Source: CAD feature listing. Evaluate the final solid. Frame: model axes, mm. Face numbers are marked on the shaded views. Give positions to 0.01 mm unless a question says otherwise; leave off trailing zeros. Order: outer loops, then holes, each group sorted by start corner. A loop starts at its lowest first (then second) coordinate and runs counter-clockwise, first axis right, second up. Notation, with made-up numbers: M 9.25,4.25 L 35.25,4.25 A23 ccw 35.25,23.25 Z; hole C -31.5,-14.75 d8. An arc over 180 degrees is marked long. Use CSV: the item, a comma, the result in double quotes. Start each with the question number.
1. Mould query, pull axis X, two halves, no side actions, for the marked faces 1, 2, 3 and 4. Classes: released by +X, released by -X, zero draft, split by the parting line, or undercut.
2. Section query A-A, the plane x = 0. Return the cut outline in (y, z), plus the area to 3 significant figures.
3. Section query C-C, the plane z = -9. Return the cut outline in (x, y).
4. Line query: line 1 along Y through (x, z) = (0, -2); line 2 along Y through (x, z) = (12, -6); line 3 along X through (y, z) = (17, 18.5). Output: solid intervals per line, ascending. Write a range as [from, to].
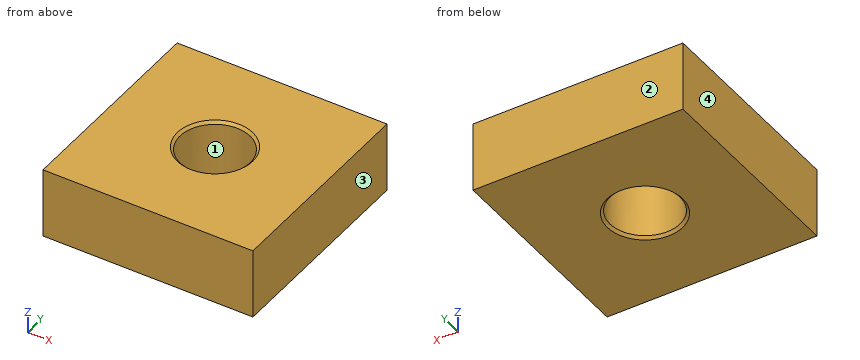
from build123d import *

# Parameters (mm, degrees)
SKETCH1_W          = 120
SKETCH1_H          = 120
SKETCH1_R          = 20
EXTRUDE1_DEPTH     = 20
FRAME_CHAMFER_SIZE = 1.5


with BuildPart() as part:
    # Sketch1 → Extrude1 (new body, symmetric)
    with BuildSketch(Plane.XY):
        Rectangle(SKETCH1_W, SKETCH1_H)
        Circle(SKETCH1_R, mode=Mode.SUBTRACT)
    extrude(amount=EXTRUDE1_DEPTH, both=True)

    # Frame Chamfer
    frame_chamfer_edges = [part.edges().sort_by_distance(p)[0] for p in [
        (-20, 0, -20),
        (-20, 0, 20),
    ]]
    chamfer(frame_chamfer_edges, length=FRAME_CHAMFER_SIZE)


solid = part.part
Result set:
1,face 1,"undercut"
1,face 2,"zero draft"
1,face 3,"released by +X"
1,face 4,"released by -X"
2,outline,"M -60,-20 L -21.5,-20 L -20,-18.5 L -20,18.5 L -21.5,20 L -60,20 Z; M 20,-18.5 L 21.5,-20 L 60,-20 L 60,20 L 21.5,20 L 20,18.5 Z"
2,area,"3,200 mm2"
3,outline,"M -60,-60 L 60,-60 L 60,60 L -60,60 Z; hole C 0,0 d40"
4,line 1,"[-60, -20], [20, 60]"
4,line 2,"[-60, -16], [16, 60]"
4,line 3,"[-60, -10.54], [10.54, 60]"
